Input: part model. Units: mm. Frame: model coordinates. Face numbers are marked on the shaded views. A direction names the side the tool comes from. Coordinates: 2 decimals unless noted, no trailing zeros. Loops run counter-clockwise (first coordinate to the right, second up) from the corner with the lowest first, then second, coordinate; pieces in that order, holes last. Notation, with made-up numbers: M 83,23 L 101,23 A23 ccw 101,61 Z; hole C 49,-29.5 d4. An arc over 180 degrees is marked long. Use a Markdown table: item, result. Add a question column.
1. Line query: L1, parallel to Z at x = -26.75, y = 10; L2, parallel to Y at x = 1, z = 3.75; L3, parallel to X at y = -4.5, z = 3.75. Output: solid intervals per line, ascending. Write a range as [from, to].
2. Section D-D on z = 5. Output: boundary loops of the cut face in (x, y), then the cut area to 3 significant figures.
3. Set-up query: the marked faces 1 and 2. Return all of +Z, -Z, +X, -X, +Y, -Y with unobstructed straight access to the full face (end or side cutting, diameter ignored); none if empty.
4. Draft query along Y for the marked faces 3, 4 and 5. Return one class per face: +Y half, -Y half, draft (parallel to the pull), parting line (faces both ways), or undercut.
5. Section C-C on y = 10. Output: boundary loops of the cut face in (x, z), then the cut area to 3 significant figures.
6. Section A-A on x = -11.5. Output: boundary loops of the cut face in (y, z), then the cut area to 3 significant figures.
7. Pin query (flat end, axial travel): pin 1 (1.5 mm diameter, centred on y = 10, z = 5, fed in from -X); pin 2 (2 mm diameter, centred on y = -10, z = 5, fed in from +X). Return the tip coordinate at first contact, or that it passes through.
8. Section B-B on x = -22. Output: boundary loops of the cut face in (y, z), then the cut area to 3 significant figures.
```python
from build123d import *

# Parameters (mm, degrees)
F0_W     = 62
F0_H     = 32
F0_W_2   = 30
F0_H_2   = 22
F1_DEPTH = 10
F2_R     = 2.1
F3_DEPTH = 10.001
F4_R     = 1.25
F5_DEPTH = 15
F6_R     = 1.25
F7_DEPTH = 15


with BuildPart() as f1:
    # F0 (on Top) → F1 (new body)
    with BuildSketch(Plane.XY):
        Rectangle(F0_W, F0_H)
        Rectangle(F0_W_2, F0_H_2, mode=Mode.SUBTRACT)
    extrude(amount=F1_DEPTH)

    # F2 (on face) → F3 (cut, through all)
    with BuildSketch(Plane.XY.offset(10)):
        with Locations((-22, 5)):
            Circle(F2_R)
        with Locations((-22, -5)):
            Circle(F2_R)
        with Locations((22, 5)):
            Circle(F2_R)
        with Locations((22, -5)):
            Circle(F2_R)
    extrude(amount=-F3_DEPTH, mode=Mode.SUBTRACT)

    # F4 (on face) → F5 (cut)
    with BuildSketch(Plane(origin=(-31, 0, 0), x_dir=(0, -1, 0), z_dir=(-1, 0, 0))):
        with Locations((10, 5)):
            Circle(F4_R)
        with Locations((-10, 5)):
            Circle(F4_R)
    extrude(amount=-F5_DEPTH, mode=Mode.SUBTRACT)

    # F6 (on face) → F7 (cut)
    with BuildSketch(Plane.YZ.offset(31)):
        with Locations((-10, 5)):
            Circle(F6_R)
        with Locations((10, 5)):
            Circle(F6_R)
    extrude(amount=-F7_DEPTH, mode=Mode.SUBTRACT)


solid = f1.part
```
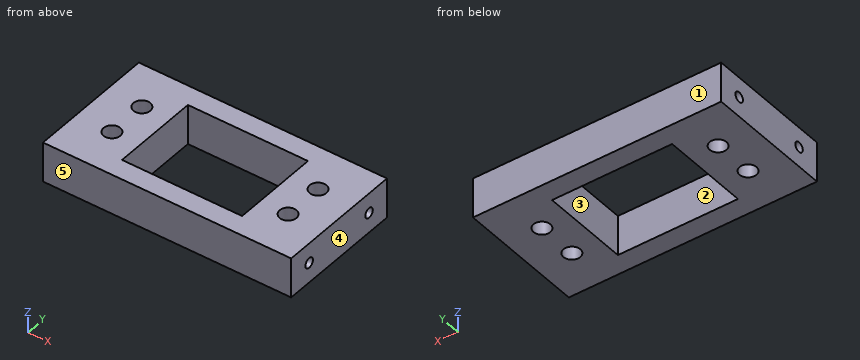
Answers below:
| question | item | result |
|---|---|---|
| 1 | L1 | z = [0, 3.75], [6.25, 10] |
| 1 | L2 | y = [-16, -11], [11, 16] |
| 1 | L3 | x = [-31, -24.04], [-19.96, -15], [15, 19.96], [24.04, 31] |
| 2 | outline | M -31,-16 L 31,-16 L 31,-11.25 L 16,-11.25 L 16,-8.75 L 31,-8.75 L 31,8.75 L 16,8.75 L 16,11.25 L 31,11.25 L 31,16 L -31,16 L -31,11.25 L -16,11.25 L -16,8.75 L -31,8.75 L -31,-8.75 L -16,-8.75 L -16,-11.25 L -31,-11.25 Z; hole C -22,-5 d4.2; hole C -22,5 d4.2; hole M -15,-11 L 15,-11 L 15,11 L -15,11 Z; hole C 22,-5 d4.2; hole C 22,5 d4.2 |
| 2 | area | 1,120 mm² |
| 3 | face 1 | +Z, -Z, +X, -X, +Y |
| 3 | face 2 | +Z, -Z |
| 4 | face 3 | undercut |
| 4 | face 4 | draft |
| 4 | face 5 | -Y half |
| 5 | outline | M -31,0 L -15,0 L -15,10 L -31,10 L -31,6.25 L -16,6.25 L -16,3.75 L -31,3.75 Z; M 15,0 L 31,0 L 31,3.75 L 16,3.75 L 16,6.25 L 31,6.25 L 31,10 L 15,10 Z |
| 5 | area | 245 mm² |
| 6 | outline | M -16,0 L -11,0 L -11,10 L -16,10 Z; M 11,0 L 16,0 L 16,10 L 11,10 Z |
| 6 | area | 100 mm² |
| 7 | pin 1 | stops at x = -16 |
| 7 | pin 2 | stops at x = 16 |
| 8 | outline | M -16,0 L -7.1,0 L -7.1,10 L -16,10 Z; M -2.9,0 L 2.9,0 L 2.9,10 L -2.9,10 Z; M 7.1,0 L 16,0 L 16,10 L 7.1,10 Z; hole C -10,5 d2.5; hole C 10,5 d2.5 |
| 8 | area | 226 mm² |
